from build123d import *

# Parameters (mm, degrees)
EXTRUDE_1_DEPTH      = 10
SKETCH_5_R           = 2.6
CUT_EXTRUDE_3_DEPTH  = 10
FILLET_5_R           = 3
FILLET_6_R           = 3
FILLET_7_R           = 3
SKETCH_7_R           = 5.5
CUT_EXTRUDE_4_DEPTH  = 5
SKETCH_12_R          = 2.553682631
CUT_EXTRUDE_9_DEPTH  = 9
EXTRUDE_2_DEPTH      = 5
CUT_EXTRUDE_START    = 5
SKETCH_14_R          = 5.5
CUT_EXTRUDE_12_DEPTH = 5
EXTRUDE_START        = 5
EXTRUDE_6_DEPTH      = 5
SKETCH_22_R          = 5.5
EXTRUDE_7_DEPTH      = 5
SKETCH_24_R          = 5.5
CUT_EXTRUDE_14_DEPTH = 3
SKETCH_25_R          = 2.65
CUT_EXTRUDE_15_DEPTH = 3
SKETCH_26_R          = 2.65
CUT_EXTRUDE_16_DEPTH = 5
SKETCH_29_R          = 2.65
EXTRUDE_8_DEPTH      = 10
EXTRUDE_START_2      = 3
SKETCH_30_R          = 5.5
EXTRUDE_9_DEPTH      = 3
CUT_EXTRUDE_18_DEPTH = 3
SKETCH_33_R          = 5.5
SKETCH_33_R_2        = 2.6
EXTRUDE_10_DEPTH     = 5
SKETCH_34_W          = 118.655960463
SKETCH_34_H          = 108.474675719
CUT_EXTRUDE_20_DEPTH = 3
CUT_EXTRUDE_21_DEPTH = 108.211729676
SKETCH_36_R          = 2.6
CUT_EXTRUDE_23_DEPTH = 108.365520444


with BuildPart() as part:
    # 草图1 → 凸台-拉伸1 (new body)
    with BuildSketch(Plane(origin=(0, 0, 0), x_dir=(1, 0, 0), z_dir=(0, 1, 0))):
        Polygon((0, 0), (0, 80), (80, 0), align=None)
    extrude(amount=EXTRUDE_1_DEPTH)

    # 草图5 → 切除-拉伸3 (cut)
    with BuildSketch(Plane(origin=(0, 10, 0), x_dir=(1, 0, 0), z_dir=(0, 1, 0))):
        with Locations(Location((6.5, 6.5, 0), (0, 0, 270))):
            Circle(SKETCH_5_R)
        with Locations(Location((6.5, 46.5, 0), (0, 0, 270))):
            Circle(SKETCH_5_R)
        with Locations(Location((46.5, 6.5, 0), (0, 0, 270))):
            Circle(SKETCH_5_R)
    extrude(amount=-CUT_EXTRUDE_3_DEPTH, mode=Mode.SUBTRACT)

    # 圆角5
    fillet_5_edges = [part.edges().sort_by_distance(p)[0] for p in [
        (80, 5, 0),
    ]]
    fillet(fillet_5_edges, radius=FILLET_5_R)

    # 圆角6
    fillet_6_edges = [part.edges().sort_by_distance(p)[0] for p in [
        (0, 5, -80),
    ]]
    fillet(fillet_6_edges, radius=FILLET_6_R)

    # 圆角7
    fillet_7_edges = [part.edges().sort_by_distance(p)[0] for p in [
        (0, 5, 0),
    ]]
    fillet(fillet_7_edges, radius=FILLET_7_R)

    # 草图7 → 切除-拉伸4 (cut)
    with BuildSketch(Plane(origin=(0, 10, 0), x_dir=(1, 0, 0), z_dir=(0, 1, 0))):
        with Locations(Location((6.5, 6.5, 0), (0, 0, 270))):
            Circle(SKETCH_7_R)
        with Locations(Location((6.5, 46.5, 0), (0, 0, 270))):
            Circle(SKETCH_7_R)
        with Locations(Location((46.5, 6.5, 0), (0, 0, 270))):
            Circle(SKETCH_7_R)
    extrude(amount=-CUT_EXTRUDE_4_DEPTH, mode=Mode.SUBTRACT)

    # 草图12 → 切除-拉伸9 (cut)
    with BuildSketch(Plane.XZ):
        with Locations((8.5, -46.5)):
            Circle(SKETCH_12_R)
    extrude(amount=-CUT_EXTRUDE_9_DEPTH, mode=Mode.SUBTRACT)

    # 草图13 → 凸台-拉伸2 (add)
    with BuildSketch(Plane.XZ):
        with BuildLine():
            ThreePointArc((7.559676255, -48.87425488), (5.946317369, -46.5), (7.559676255, -44.12574512))
            ThreePointArc((7.559676255, -44.12574512), (3.9, -46.5), (7.559676255, -48.87425488))
        make_face()
    extrude(amount=-EXTRUDE_2_DEPTH)

    # 草图14 → 切除-拉伸12 (cut)
    with BuildSketch(Plane(origin=(0, 5, 0), x_dir=(1, 0, 0), z_dir=(0, 1, 0)).offset(CUT_EXTRUDE_START)):
        with Locations((8.5, 46.5)):
            Circle(SKETCH_14_R)
        with Locations((6.5, 46.5)):
            Circle(SKETCH_14_R)
    extrude(amount=-CUT_EXTRUDE_12_DEPTH, mode=Mode.SUBTRACT)

    # 草图21 → 凸台-拉伸6 (add)
    with BuildSketch(Plane(origin=(0, 5, 0), x_dir=(1, 0, 0), z_dir=(0, 1, 0)).offset(EXTRUDE_START)):
        with BuildLine():
            ThreePointArc((7.5, 41.091673087), (3, 46.5), (7.5, 51.908326913))
            ThreePointArc((7.5, 51.908326913), (1, 46.5), (7.5, 41.091673087))
        make_face()
    extrude(amount=-EXTRUDE_6_DEPTH)

    # 草图22 → 凸台-拉伸7 (add)
    with BuildSketch(Plane(origin=(0, 5, 0), x_dir=(1, 0, 0), z_dir=(0, 1, 0)).offset(EXTRUDE_START)):
        with Locations((8.5, 46.5)):
            Circle(SKETCH_22_R)
    extrude(amount=-EXTRUDE_7_DEPTH)

    # 草图24 → 切除-拉伸14 (cut)
    with BuildSketch(Plane(origin=(0, 10, 0), x_dir=(1, 0, 0), z_dir=(0, 1, 0))):
        with Locations(Location((8.5, 46.5, 0), (0, 0, 270))):
            Circle(SKETCH_24_R)
    extrude(amount=-CUT_EXTRUDE_14_DEPTH, mode=Mode.SUBTRACT)

    # 草图25 → 切除-拉伸15 (cut)
    with BuildSketch(Plane.XZ.offset(-5)):
        with Locations(Location((8.5, -46.5, 0), (0, 0, 270))):
            Circle(SKETCH_25_R)
    extrude(amount=-CUT_EXTRUDE_15_DEPTH, mode=Mode.SUBTRACT)

    # 草图26 → 切除-拉伸16 (cut)
    with BuildSketch(Plane.XZ):
        with Locations(Location((8.5, -46.5, 0), (0, 0, 270))):
            Circle(SKETCH_26_R)
    extrude(amount=-CUT_EXTRUDE_16_DEPTH, mode=Mode.SUBTRACT)

    # 草图29 → 凸台-拉伸8 (add)
    with BuildSketch(Plane.XZ):
        with Locations(Location((8.5, -46.5, 0), (0, 0, 270))):
            Circle(SKETCH_29_R)
    extrude(amount=-EXTRUDE_8_DEPTH)

    # 草图30 → 凸台-拉伸9 (add)
    with BuildSketch(Plane(origin=(0, 7, 0), x_dir=(1, 0, 0), z_dir=(0, 1, 0)).offset(EXTRUDE_START_2)):
        with Locations((8.5, 46.5)):
            Circle(SKETCH_30_R)
    extrude(amount=-EXTRUDE_9_DEPTH)

    # 草图2 → 切除-拉伸18 (cut)
    with BuildSketch(Plane.XZ):
        with BuildLine():
            ThreePointArc((6.5, -56.5), (8.413417162, -56.880602337), (10.035533906, -57.964466094))
            Line((10.035533906, -57.964466094), (57.964466094, -10.035533906))
            ThreePointArc((57.964466094, -10.035533906), (56.880602337, -8.413417162), (56.5, -6.5))
            Line((56.5, -6.5), (54.428932188, -6.5))
            Line((54.428932188, -6.5), (6.5, -54.428932188))
            Line((6.5, -54.428932188), (6.5, -56.5))
        make_face()
        with BuildLine():
            Line((57.964466094, -10.035533906), (10.035533906, -57.964466094))
            ThreePointArc((10.035533906, -57.964466094), (11.119397663, -59.586582838), (11.5, -61.5))
            ThreePointArc((11.5, -61.5), (11.119397663, -63.413417162), (10.035533906, -65.035533906))
            Line((10.035533906, -65.035533906), (65.035533906, -10.035533906))
            ThreePointArc((65.035533906, -10.035533906), (61.5, -11.5), (57.964466094, -10.035533906))
        make_face()
        with BuildLine():
            Line((6.5, -66.5), (6.5, -61.5))
            Line((6.5, -61.5), (6.5, -56.5))
            ThreePointArc((6.5, -56.5), (4.586582838, -56.880602337), (2.964466094, -57.964466094))
            ThreePointArc((2.964466094, -57.964466094), (1.880602337, -63.413417162), (6.5, -66.5))
        make_face()
        with BuildLine():
            Line((6.5, -56.5), (6.5, -61.5))
            Line((6.5, -61.5), (10.035533906, -57.964466094))
            ThreePointArc((10.035533906, -57.964466094), (8.413417162, -56.880602337), (6.5, -56.5))
        make_face()
        with BuildLine():
            Line((10.035533906, -57.964466094), (6.5, -61.5))
            Line((6.5, -61.5), (6.5, -66.5))
            ThreePointArc((6.5, -66.5), (8.413417162, -66.119397663), (10.035533906, -65.035533906))
            ThreePointArc((10.035533906, -65.035533906), (11.119397663, -63.413417162), (11.5, -61.5))
            ThreePointArc((11.5, -61.5), (11.119397663, -59.586582838), (10.035533906, -57.964466094))
        make_face()
        with BuildLine():
            Line((6.5, -56.5), (6.5, -61.5))
            Line((6.5, -61.5), (10.035533906, -57.964466094))
            ThreePointArc((10.035533906, -57.964466094), (8.413417162, -56.880602337), (6.5, -56.5))
        make_face()
        with BuildLine():
            Line((10.035533906, -57.964466094), (6.5, -61.5))
            Line((6.5, -61.5), (6.5, -66.5))
            ThreePointArc((6.5, -66.5), (8.413417162, -66.119397663), (10.035533906, -65.035533906))
            ThreePointArc((10.035533906, -65.035533906), (11.119397663, -63.413417162), (11.5, -61.5))
            ThreePointArc((11.5, -61.5), (11.119397663, -59.586582838), (10.035533906, -57.964466094))
        make_face()
        with BuildLine():
            ThreePointArc((2.964466094, -57.964466094), (4.586582838, -56.880602337), (6.5, -56.5))
            Line((6.5, -56.5), (6.5, -54.428932188))
            Line((6.5, -54.428932188), (2.964466094, -57.964466094))
        make_face()
        with BuildLine():
            Line((54.428932188, -6.5), (56.5, -6.5))
            ThreePointArc((56.5, -6.5), (56.880602337, -4.586582838), (57.964466094, -2.964466094))
            Line((57.964466094, -2.964466094), (54.428932188, -6.5))
        make_face()
        with BuildLine():
            Line((56.5, -6.5), (61.5, -6.5))
            Line((61.5, -6.5), (66.5, -6.5))
            ThreePointArc((66.5, -6.5), (63.413417162, -1.880602337), (57.964466094, -2.964466094))
            ThreePointArc((57.964466094, -2.964466094), (56.880602337, -4.586582838), (56.5, -6.5))
        make_face()
        with BuildLine():
            ThreePointArc((56.5, -6.5), (56.880602337, -8.413417162), (57.964466094, -10.035533906))
            Line((57.964466094, -10.035533906), (61.5, -6.5))
            Line((61.5, -6.5), (56.5, -6.5))
        make_face()
        with BuildLine():
            Line((61.5, -6.5), (57.964466094, -10.035533906))
            ThreePointArc((57.964466094, -10.035533906), (61.5, -11.5), (65.035533906, -10.035533906))
            ThreePointArc((65.035533906, -10.035533906), (66.119397663, -8.413417162), (66.5, -6.5))
            Line((66.5, -6.5), (61.5, -6.5))
        make_face()
        with BuildLine():
            ThreePointArc((56.5, -6.5), (56.880602337, -8.413417162), (57.964466094, -10.035533906))
            Line((57.964466094, -10.035533906), (61.5, -6.5))
            Line((61.5, -6.5), (56.5, -6.5))
        make_face()
        with BuildLine():
            Line((61.5, -6.5), (57.964466094, -10.035533906))
            ThreePointArc((57.964466094, -10.035533906), (61.5, -11.5), (65.035533906, -10.035533906))
            ThreePointArc((65.035533906, -10.035533906), (66.119397663, -8.413417162), (66.5, -6.5))
            Line((66.5, -6.5), (61.5, -6.5))
        make_face()
    extrude(amount=-CUT_EXTRUDE_18_DEPTH, mode=Mode.SUBTRACT)

    # 草图33 → 凸台-拉伸10 (add)
    # profile 1 of 2: a face of its own
    with BuildSketch(Plane(origin=(0, 10, 0), x_dir=(1, 0, 0), z_dir=(0, 1, 0))):
        with Locations((6.5, 6.5)):
            Circle(SKETCH_33_R)
        with Locations(Location((6.5, 6.5, 0), (0, 0, 270))):
            Circle(SKETCH_33_R_2, mode=Mode.SUBTRACT)
    # profile 2 of 2: a face of its own
    with BuildSketch(Plane(origin=(0, 10, 0), x_dir=(1, 0, 0), z_dir=(0, 1, 0))):
        with Locations((46.5, 6.5)):
            Circle(SKETCH_33_R)
        with Locations(Location((46.5, 6.5, 0), (0, 0, 270))):
            Circle(SKETCH_33_R_2, mode=Mode.SUBTRACT)
    extrude(amount=-EXTRUDE_10_DEPTH)

    # 草图34 → 切除-拉伸20 (cut)
    with BuildSketch(Plane(origin=(0, 10, 0), x_dir=(1, 0, 0), z_dir=(0, 1, 0))):
        with Locations((37.4387476, 33.290816779)):
            Rectangle(SKETCH_34_W, SKETCH_34_H)
    extrude(amount=-CUT_EXTRUDE_20_DEPTH, mode=Mode.SUBTRACT)

    # 草图35 → 切除-拉伸21 (cut, through all)
    with BuildSketch(Plane.XZ.offset(-3)):
        with BuildLine():
            Line((8.267766953, -63.267766953), (63.267766953, -8.267766953))
            ThreePointArc((63.267766953, -8.267766953), (63.267766953, -4.732233047), (59.732233047, -4.732233047))
            Line((59.732233047, -4.732233047), (4.732233047, -59.732233047))
            ThreePointArc((4.732233047, -59.732233047), (4.732233047, -63.267766953), (8.267766953, -63.267766953))
        make_face()
    extrude(amount=-CUT_EXTRUDE_21_DEPTH, mode=Mode.SUBTRACT)

    # 草图36 → 切除-拉伸23 (cut, through all)
    with BuildSketch(Plane(origin=(0, 7, 0), x_dir=(1, 0, 0), z_dir=(0, 1, 0))):
        with Locations(Location((6.5, 46.5, 0), (0, 0, 270))):
            Circle(SKETCH_36_R)
    extrude(amount=-CUT_EXTRUDE_23_DEPTH, mode=Mode.SUBTRACT)


solid = part.part
Design review of the part built by this model. Coordinates are the model's own, in mm. A direction names the side the tool comes from. Coordinates: 2 decimals unless noted, no trailing zeros. Order: outer loops, then holes, each group sorted by start corner. A loop starts at its lowest first (then second) coordinate and runs counter-clockwise, first axis right, second up. Notation, with made-up numbers: (-16, 55) -> (-6, 55) arc R32 ccw to (-6, 85) -> close; hole circle Ø10 at (-25.75, 71.5). An arc over 180 degrees is marked (long way). Use one line per item in the form item = value. Start each with the question number.
(1) Add section C-C on z = -37.5. State the section outline as (x, y) points, plus the area to 3 significant figures.
(2) Add section D-D on z = -46.5. State the section outline as (x, y) points.
(3) For faces 4 (the flat face through (21, 0, -21)), 5 (the flat face through (35.383, 4.972, -36.153)), 6 (the flat face through (30.85, 1.48, -30.08)), list the 3-axis set-ups (+Z, -Z, +X, -X, +Y, -Y) from which the entire face can be reached by the end or side of a thin tool; tool diameter is ignored.
(4) For probe 1 along X at (y, z) = (5.75, -6.5); probe 2 along Z at (x, y) = (46, 6.25); probe 3 along Z at (x, y) = (45, 4.75), list the stretches that pass through material, from the lowest coordinate up.
(5) The part is to be moulded in two halves that separate along X. For faces 1 (the flat face through (0, 3, -37)), 2 (the flat face through (36, 3, -36)), 3 (the cylindrical face through (1.81, 3.55, -75.51)), say which applies: +X half, -X half, draft (parallel to the pull), parting line (faces both ways), or undercut.
(6) Insertion check: pin 1 (4.5 mm diameter, centred on x = 46.5, z = -6.5, fed in from +Y); pin 2 (2 mm diameter, centred on y = 2.5, z = -39.5, fed in from +X). Each pin has a flat end and moves straight along its axis. Give the tip position at first contact, or say it passes through.
(7) Add section A-A on y = 5. State the section outline as (x, z) points, plus the area to 3 significant figures.
(8) Add section B-B on x = 11.5. State the section outline as (y, z) points.
Answer block:
q1.outline = (0, 0) -> (23.43, 0) -> (23.43, 3) -> (26.96, 3) -> (26.96, 7) -> (0, 7) -> close; (34.04, 3) -> (37.57, 3) -> (37.57, 0) -> (42.5, 0) -> (42.5, 7) -> (34.04, 7) -> close
q1.area = 227 mm²
q2.outline = (0, 0) -> (3.9, 0) -> (3.9, 7) -> (0, 7) -> close; (9.1, 0) -> (14.43, 0) -> (14.43, 3) -> (17.96, 3) -> (17.96, 7) -> (9.1, 7) -> close; (25.04, 3) -> (28.57, 3) -> (28.57, 0) -> (33.5, 0) -> (33.5, 7) -> (25.04, 7) -> close
q3.face_4 = +Z, -Z, +X, -X, -Y
q3.face_5 = +Y, -Y
q3.face_6 = -Y
q4.probe_1 = 0 to 3.9, 9.1 to 43.9, 49.1 to 57.96, 64 to 73.5
q4.probe_2 = -34 to -25.54, -18.46 to -9.05, -3.95 to 0
q4.probe_3 = -35 to -26.54, -19.46 to -8.62, -4.38 to 0
q5.face_1 = -X half
q5.face_2 = undercut
q5.face_3 = parting line
q6.pin_1 = through
q6.pin_2 = 41.5
q7.outline = (0, -72.76) arc R3 ccw to (5.12, -74.88) -> (74.88, -5.12) arc R3 ccw to (72.76, 0) -> (3, 0) arc R3 ccw to (0, -3) -> close; hole circle Ø5.2 at (6.5, -46.5); hole circle Ø5.2 at (6.5, -6.5); hole (4.73, -59.73) arc R2.5 ccw to (8.27, -63.27) -> (63.27, -8.27) arc R2.5 ccw to (59.73, -4.73) -> close; hole circle Ø5.2 at (46.5, -6.5)
q7.area = 2,700 mm²
q8.outline = (0, -68.5) -> (7, -68.5) -> (7, -60.04) -> (3, -60.04) -> (3, -63.57) -> (0, -63.57) -> close; (0, -49.43) -> (3, -49.43) -> (3, -52.96) -> (7, -52.96) -> (7, 0) -> (0, 0) -> close
